Source: CAD feature listing. Evaluate the final solid. Frame: model axes, mm. A direction names the side the tool comes from. Give positions to 0.01 mm unless a question says otherwise; leave off trailing zeros. Order: outer loops, then holes, each group sorted by start corner. A loop starts at its lowest first (then second) coordinate and runs counter-clockwise, first axis right, second up. Notation, with made-up numbers: M 35.25,59.5 L 47.25,59.5 A34 cw 47.25,92.5 Z; hole C -39.75,49 d1. An arc over 180 degrees is marked long. Answer as a JSON object with one key per item and string values. Group by question number.
1. Set-up query: faces 4 (the cylindrical face through (-38.56, 2.465, 148.814)), 5 (the cylindrical face through (-21.078, 2.465, -1.208)). Return all of +Z, -Z, +X, -X, +Y, -Y with unobstructed straight access to the full face (end or side cutting, diameter ignored); none if empty.
2. Section query D-D (y = 0.75). Count the separate pieces of the cut face and the enclosed holes in it, plus the area to 3 significant figures.
3. Section query C-C (x = 188). Output: boundary loops of the cut face in (y, z), plus the area to 3 significant figures.
4. Section query A-A (x = 51). Output: boundary loops of the cut face in (y, z).
5. Material intervals for L1, parallel to Z at x = 218, y = 2; L2, parallel to X at y = 0.6, z = 109.5; L3, parallel to Z at x = 89, y = 3.7, sorted ascending. Write a range as [from, to].
6. Section query B-B (z = 76). Output: boundary loops of the cut face in (x, y).
7. Pull-direction query (X, two-part tool) for faces 1 (the cylindrical face through (-22, 2, 130)), 2 (the flat face through (189, 5, 63)), 3 (the cylindrical face through (-39.42, 2.46, -18.22)); classes: +X half, -X half, draft (parallel to the pull), parting line (faces both ways), or undercut.
8. Pin query (flat end, axial travel): P1, Ø1.5, axis at y = 3, z = 115, coming from the -X side; P2, Ø2.5, axis at x = 229, y = 3, coming from the +Z side; P3, Ø1.5, axis at y = 2, z = 13.5, coming from the -X side. Return the tip coordinate at first contact, or that it passes through.
from build123d import *

# Parameters (mm, degrees)
SKETCH1_R           = 1.375
SKETCH1_R_2         = 1.318565094
BOSS_EXTRUDE1_DEPTH = 5


with BuildPart() as part:
    # Sketch1 → Boss-Extrude1 (new body)
    with BuildSketch(Plane(origin=(0, 0, 0), x_dir=(1, 0, 0), z_dir=(0, 1, 0))):
        with BuildLine():
            Line((279.931043908, -90.367567702), (279.931043908, -109.497567702))
            ThreePointArc((279.931043908, -109.497567702), (263.821916873, -148.388440667), (224.931043908, -164.497567702))
            Line((224.931043908, -164.497567702), (-0.098956092, -164.497567702))
            ThreePointArc((-0.098956092, -164.497567702), (-38.989829057, -148.388440667), (-55.098956092, -109.497567702))
            Line((-55.098956092, -109.497567702), (-55.098956092, -20.237567702))
            ThreePointArc((-55.098956092, -20.237567702), (-38.989829057, 18.653305263), (-0.098956092, 34.762432298))
            Line((-0.098956092, 34.762432298), (224.931043908, 34.762432298))
            ThreePointArc((224.931043908, 34.762432298), (263.821916873, 18.653305263), (279.931043908, -20.237567702))
            Line((279.931043908, -20.237567702), (279.931043908, -39.367567702))
            ThreePointArc((279.931043908, -39.367567702), (279.052364252, -37.246247359), (276.931043908, -36.367567702))
            Line((276.931043908, -36.367567702), (255.431043908, -36.367567702))
            Line((255.431043908, -36.367567702), (255.431043908, -40.367567702))
            ThreePointArc((255.431043908, -40.367567702), (254.552364252, -42.488888046), (252.431043908, -43.367567702))
            Line((252.431043908, -43.367567702), (251.431043908, -43.367567702))
            ThreePointArc((251.431043908, -43.367567702), (249.309723565, -42.488888046), (248.431043908, -40.367567702))
            Line((248.431043908, -40.367567702), (248.431043908, -36.367567702))
            Line((248.431043908, -36.367567702), (200.931043908, -36.367567702))
            Line((200.931043908, -36.367567702), (200.931043908, -40.367567702))
            ThreePointArc((200.931043908, -40.367567702), (200.052364252, -42.488888046), (197.931043908, -43.367567702))
            Line((197.931043908, -43.367567702), (193.931043908, -43.367567702))
            Line((193.931043908, -43.367567702), (193.931043908, -86.867567702))
            Line((193.931043908, -86.867567702), (197.397932751, -86.867567702))
            ThreePointArc((197.397932751, -86.867567702), (199.519253094, -87.746247359), (200.397932751, -89.867567702))
            Line((200.397932751, -89.867567702), (200.397932751, -93.367567702))
            Line((200.397932751, -93.367567702), (248.431043908, -93.367567702))
            Line((248.431043908, -93.367567702), (248.431043908, -89.367567702))
            ThreePointArc((248.431043908, -89.367567702), (249.309723565, -87.246247359), (251.431043908, -86.367567702))
            Line((251.431043908, -86.367567702), (252.431043908, -86.367567702))
            ThreePointArc((252.431043908, -86.367567702), (254.552364252, -87.246247359), (255.431043908, -89.367567702))
            Line((255.431043908, -89.367567702), (255.431043908, -93.367567702))
            Line((255.431043908, -93.367567702), (276.931043908, -93.367567702))
            ThreePointArc((276.931043908, -93.367567702), (279.052364252, -92.488888046), (279.931043908, -90.367567702))
        make_face()
        with Locations(Location((251.931043908, -39.867567702, 0), (0, 0, 270))):
            Circle(SKETCH1_R, mode=Mode.SUBTRACT)
        with Locations(Location((251.931043908, -89.867567702, 0), (0, 0, 270))):
            Circle(SKETCH1_R, mode=Mode.SUBTRACT)
        with Locations(Location((197.397932751, -89.867567702, 0), (0, 0, 270))):
            Circle(SKETCH1_R_2, mode=Mode.SUBTRACT)
        with Locations(Location((197.431043908, -39.867567702, 0), (0, 0, 270))):
            Circle(SKETCH1_R, mode=Mode.SUBTRACT)
        with BuildLine():
            Line((-0.098956092, -139.497567702), (224.931043908, -139.497567702))
            ThreePointArc((224.931043908, -139.497567702), (242.734133528, -133.643996009), (253.589779051, -118.367567702))
            Line((253.589779051, -118.367567702), (251.931043908, -118.367567702))
            Line((251.931043908, -118.367567702), (175.397932751, -118.367567702))
            Line((175.397932751, -118.367567702), (175.397932751, -111.867567702))
            Line((175.397932751, -111.867567702), (168.931043908, -111.867567702))
            Line((168.931043908, -111.867567702), (168.931043908, -18.367567702))
            Line((168.931043908, -18.367567702), (175.931043908, -18.367567702))
            Line((175.931043908, -18.367567702), (175.931043908, -11.367567702))
            Line((175.931043908, -11.367567702), (251.931043908, -11.367567702))
            Line((251.931043908, -11.367567702), (253.589779051, -11.367567702))
            ThreePointArc((253.589779051, -11.367567702), (242.734133528, 3.908860605), (224.931043908, 9.762432298))
            Line((224.931043908, 9.762432298), (-0.098956092, 9.762432298))
            ThreePointArc((-0.098956092, 9.762432298), (-21.312159527, 0.975635734), (-30.098956092, -20.237567702))
            Line((-30.098956092, -20.237567702), (-30.098956092, -109.497567702))
            ThreePointArc((-30.098956092, -109.497567702), (-21.312159527, -130.710771138), (-0.098956092, -139.497567702))
        make_face(mode=Mode.SUBTRACT)
    extrude(amount=BOSS_EXTRUDE1_DEPTH)


solid = part.part
Answer sheet:
{
 "1": {"face 4": "+Z, -X, +Y, -Y", "face 5": "+Y, -Y"},
 "2": {"separate pieces": "1", "enclosed holes": "5", "area": "26,700 mm^2"},
 "3": {"outline": "M 0,-34.76 L 5,-34.76 L 5,-9.76 L 0,-9.76 Z; M 0,11.37 L 5,11.37 L 5,118.37 L 0,118.37 Z; M 0,139.5 L 5,139.5 L 5,164.5 L 0,164.5 Z", "area": "785 mm^2"},
 "4": {"outline": "M 0,-34.76 L 5,-34.76 L 5,-9.76 L 0,-9.76 Z; M 0,139.5 L 5,139.5 L 5,164.5 L 0,164.5 Z"},
 "5": {"L1": "[-34.76, -9.76], [11.37, 36.37], [93.37, 118.37], [139.5, 164.5]", "L2": "[-55.1, -30.1], [168.93, 279.93]", "L3": "[-34.76, -9.76], [139.5, 164.5]"},
 "6": {"outline": "M -55.1,0 L -30.1,0 L -30.1,5 L -55.1,5 Z; M 168.93,0 L 193.93,0 L 193.93,5 L 168.93,5 Z"},
 "7": {"face 1": "undercut", "face 2": "draft", "face 3": "-X half"},
 "8": {"P1": "x = -54.89", "P2": "z = 164.43", "P3": "x = -54.77"}
}
